CAD build for the part. Positions are in the model's coordinates, mm. A direction names the side the tool comes from. Coordinates: 2 decimals unless noted, no trailing zeros. Order: outer loops, then holes, each group sorted by start corner. A loop starts at its lowest first (then second) coordinate and runs counter-clockwise, first axis right, second up. Notation, with made-up numbers: (-16.5, 51.25) - (-8.5, 51.25) arc R21 cw to (-8.5, 74.25) - close; hole circle Ø3 at (77.5, 38.5). An arc over 180 degrees is marked (long way). Return JSON: item names as keys, results as strings.
from build123d import *

# Parameters (mm, degrees)
BOX_W          = 75
BOX_H          = 150
BOX_DEPTH      = 75
CYLINDER_R     = 30
CYLINDER_DEPTH = 150
BOX001_W       = 35
BOX001_H       = 130
BOX001_DEPTH   = 35
BOX002_W       = 50
BOX002_H       = 130
BOX002_DEPTH   = 35


with BuildPart() as part:
    # Box → Box (join)
    with BuildSketch(Plane.XY):
        with Locations((37.5, 75)):
            Rectangle(BOX_W, BOX_H)
    extrude(amount=BOX_DEPTH)

    # Cylinder → Cylinder (cut)
    with BuildSketch(Plane(origin=(37.5, 150, 37.5), x_dir=(1, 0, 0), z_dir=(0, -1, 0))):
        Circle(CYLINDER_R)
    extrude(amount=CYLINDER_DEPTH, mode=Mode.SUBTRACT)

    # Box001 → Box001 (cut)
    with BuildSketch(Plane(origin=(20, 10, 40), x_dir=(1, 0, 0), z_dir=(0, 0, 1))):
        with Locations((17.5, 65)):
            Rectangle(BOX001_W, BOX001_H)
    extrude(amount=BOX001_DEPTH, mode=Mode.SUBTRACT)

    # Box002 → Box002 (cut)
    with BuildSketch(Plane(origin=(0, 10, 0), x_dir=(1, 0, 0), z_dir=(0, 0, 1))):
        with Locations((25, 65)):
            Rectangle(BOX002_W, BOX002_H)
    extrude(amount=BOX002_DEPTH, mode=Mode.SUBTRACT)


solid = part.part
Item 1: Wall check: L1, parallel to X at y = 109, z = 37; L2, parallel to X at y = 15, z = 71; L3, parallel to Z at x = 17, y = 9. Give the ranges that are in metal, low to high. Write a range as [from, to].
Findings below:
{"L1": "x = [0, 7.5], [67.5, 75]", "L2": "x = [0, 20], [55, 75]", "L3": "z = [0, 15.6], [59.4, 75]"}
Item 2: Band-saw the part on D-D, the plane x = 59.5. List the corners of the cut face in (y, z).
Findings below:
{"outline": "(0, 0) - (150, 0) - (150, 17.1) - (0, 17.1) - close; (0, 57.9) - (150, 57.9) - (150, 75) - (0, 75) - close"}
Item 3: Band-saw the part on B-B, the plane z = 37.5. List the corners of the cut face in (x, y).
Findings below:
{"outline": "(0, 0) - (7.5, 0) - (7.5, 150) - (0, 150) - close; (67.5, 0) - (75, 0) - (75, 150) - (67.5, 150) - close"}
Item 4: Band-saw the part on C-C, the plane x = 37.5. List the corners of the cut face in (y, z).
Findings below:
{"outline": "(0, 0) - (10, 0) - (10, 7.5) - (0, 7.5) - close; (0, 67.5) - (10, 67.5) - (10, 75) - (0, 75) - close; (140, 0) - (150, 0) - (150, 7.5) - (140, 7.5) - close; (140, 67.5) - (150, 67.5) - (150, 75) - (140, 75) - close"}
Item 5: Drop flat-ended pins along their axis: P1, Ø12, axis at y = 44, z = 11.5, coming from the -X side; P2, Ø1.5, axis at y = 133.5, z = 14.5, coming from the -X side; P3, Ø8.5, axis at x = 4.5, y = 74, coming from the -Z side. Give the stop position or say it passes through.
Findings below:
{"P1": "stops at x = 50", "P2": "stops at x = 55.83", "P3": "stops at z = 35"}
Item 6: Which spindle directions (+Z, -Z, +X, -X, +Y, -Y) get a long thin tool onto all of the face, cutting with end or side? Do faces 5 (the flat face through (19, 140, 9)), 6 (the flat face through (55, 74, 68)), 7 (the flat face through (50, 74, 5)). Say none if no direction does.
Findings below:
{"face 5": "-Z, -X", "face 6": "+Z", "face 7": "+Z, -Z, -X"}
Item 7: Mould opens along X. For faces 1 (the flat face through (20, 74, 68)), 2 (the flat face through (62, 76, 75)), 3 (the flat face through (75, 74, 37)), 4 (the flat face through (0, 74, 45)) say: released by +X, released by -X, zero draft, split by the parting line, or undercut.
Findings below:
{"face 1": "undercut", "face 2": "zero draft", "face 3": "released by +X", "face 4": "released by -X"}
Item 8: Band-saw the part on A-A, the plane y = 91.5. List the corners of the cut face in (x, z), then the cut area to 3 significant figures.
Findings below:
{"outline": "(0, 35) - (7.6, 35) arc R30 cw to (20, 61.87) - (20, 75) - (0, 75) - close; (50, 0) - (75, 0) - (75, 75) - (55, 75) - (55, 61.87) arc R30 cw to (50, 10.23) - close", "area": "1,690 mm²"}
